Geometry: final body of the model. Coordinates: model frame, mm. A direction names the side the tool comes from. Give positions to 0.01 mm unless a question says otherwise; leave off trailing zeros. Order: outer loops, then holes, each group sorted by start corner. A loop starts at its lowest first (then second) coordinate and runs counter-clockwise, first axis right, second up. Notation, with made-up numbers: (61.5, -14) - (92.5, -14) arc R21 ccw to (92.5, 18) - close; hole circle Ø7 at (33.25, -5). An arc over 180 degrees is marked (long way). Put each result on its own line as item: value. Start each with the question number.
1. Section B-B on x = 4.65. Return the cut outline in (y, z), plus the area to 3 significant figures.
2. Ray query, line 1 along Y through (x, z) = (0, 0.9); line 2 along Z through (x, y) = (1.25, 1.25); line 3 along Z through (x, y) = (0.5, 4.25). Return the intervals inside material, ascending. Write a range as from..to.
3. Set-up query: faces 5 (the flat face through (-1, -1, 1.1)), 6 (the flat face through (1.9, 5, 1)), 7 (the flat face through (-1, -1, 1.33)), 8 (the flat face through (1.9, -5, 1)). Return all of +Z, -Z, +X, -X, +Y, -Y with unobstructed straight access to the full face (end or side cutting, diameter ignored); none if empty.
4. Mould query, pull axis Y, two halves, no side actions, for faces 1 (the flat face through (-1.9, -5, 1)), 2 (the cylindrical face through (-10.94, -1.79, 0.66)), 3 (the cylindrical face through (0, 8.4, 0.7)), 4 (the cylindrical face through (-8.221, 0.135, 0.674)). Classes: pulls with the +Y half, pulls with the -Y half, needs draft (parallel to the pull), parting line crosses it, or undercut.
5. First-contact query: P1, Ø2, axis at x = -4.5, z = 3, coming from the -Y side; P2, Ø4, axis at x = 0, y = 0, coming from the -Z side; P3, Ø1.5, axis at y = 5.5, z = 0.5, coming from the -X side; P4, Ø1.5, axis at x = -9, z = 0.5, coming from the -Y side. Flat tips, straight axial feed; report the tip coordinate or a pass-through.
6. Section A-A on z = 0.8. Count the separate pieces of the cut face and the enclosed holes in it, plus the area to 3 significant figures.
7. Section C-C on z = 3.3. Return the cut outline in (x, y), plus the area to 3 significant figures.
from build123d import *

# Parameters (mm, degrees)
AUFSATZ_LINEAR_AUSTRAGEN1_DEPTH      = 1.33
SKIZZE2_R                            = 3.4
SKIZZE2_R_2                          = 2.3
AUFSATZ_LINEAR_AUSTRAGEN2_DEPTH      = 2.3
AUFSATZ_LINEAR_AUSTRAGEN2_DEPTH_BACK = 1.33
SKIZZE3_R                            = 1.25
SCHNITT_LINEAR_AUSTRAGEN1_DEPTH      = 2.33
SKIZZE4_R                            = 2.35
SCHNITT_LINEAR_AUSTRAGEN2_DEPTH      = 1.1
SKIZZE5_R                            = 0.45
SCHNITT_LINEAR_AUSTRAGEN3_DEPTH      = 2.33
SKIZZE7_W                            = 8.843573308
SKIZZE7_H                            = 7.939116947
SKIZZE7_W_2                          = 8.543023068
SKIZZE7_H_2                          = 6.617341639
SCHNITT_LINEAR_AUSTRAGEN4_DEPTH      = 1.33
VERRUNDUNG1_R                        = 2


with BuildPart() as part:
    # Skizze1 → Aufsatz-Linear austragen1 (new body)
    with BuildSketch(Plane.XY):
        with BuildLine():
            Line((-16.79191458, 1.869621687), (-1.9, 3))
            Line((-1.9, 3), (-1.9, 6.5))
            ThreePointArc((-1.9, 6.5), (0, 8.4), (1.9, 6.5))
            Line((1.9, 6.5), (1.9, 3))
            Line((1.9, 3), (16.79191458, 1.869621687))
            ThreePointArc((16.79191458, 1.869621687), (18.525, 0), (16.79191458, -1.869621687))
            Line((16.79191458, -1.869621687), (1.9, -3))
            Line((1.9, -3), (1.9, -6.5))
            ThreePointArc((1.9, -6.5), (0, -8.4), (-1.9, -6.5))
            Line((-1.9, -6.5), (-1.9, -3))
            Line((-1.9, -3), (-16.79191458, -1.869621687))
            ThreePointArc((-16.79191458, -1.869621687), (-18.525, 0), (-16.79191458, 1.869621687))
        make_face()
    extrude(amount=AUFSATZ_LINEAR_AUSTRAGEN1_DEPTH)

    # Skizze2 → Aufsatz-Linear austragen2 (add, two sides)
    with BuildSketch(Plane.XY.offset(1.33)) as aufsatz_linear_austragen2_sk:
        Circle(SKIZZE2_R)
        Circle(SKIZZE2_R_2, mode=Mode.SUBTRACT)
    extrude(amount=AUFSATZ_LINEAR_AUSTRAGEN2_DEPTH)
    extrude(aufsatz_linear_austragen2_sk.sketch, amount=-AUFSATZ_LINEAR_AUSTRAGEN2_DEPTH_BACK)

    # Skizze3 → Schnitt-Linear austragen1 (cut, through all)
    with BuildSketch(Plane.XY.offset(1.33)):
        Circle(SKIZZE3_R)
    extrude(amount=-SCHNITT_LINEAR_AUSTRAGEN1_DEPTH, mode=Mode.SUBTRACT)

    # Skizze4 → Schnitt-Linear austragen2 (cut)
    with BuildSketch(Plane(origin=(0, 0, 0), x_dir=(-1, 0, 0), z_dir=(0, 0, -1))):
        Circle(SKIZZE4_R)
    extrude(amount=-SCHNITT_LINEAR_AUSTRAGEN2_DEPTH, mode=Mode.SUBTRACT)

    # Skizze5 → Schnitt-Linear austragen3 (cut, through all)
    with BuildSketch(Plane.XY.offset(1.33)):
        with Locations((0, 6.5)):
            Circle(SKIZZE5_R)
        with Locations((-16.65, 0)):
            Circle(SKIZZE5_R)
        with Locations((0, 4.5)):
            Circle(SKIZZE5_R)
        with Locations((-14.65, 0)):
            Circle(SKIZZE5_R)
        with Locations((-12.65, 0)):
            Circle(SKIZZE5_R)
        with Locations((-10.65, 0)):
            Circle(SKIZZE5_R)
        with Locations((-8.65, 0)):
            Circle(SKIZZE5_R)
        with Locations((-6.65, 0)):
            Circle(SKIZZE5_R)
        with Locations((-4.65, 0)):
            Circle(SKIZZE5_R)
        with Locations((0, -4.5)):
            Circle(SKIZZE5_R)
        with Locations((0, -6.5)):
            Circle(SKIZZE5_R)
        with Locations((4.65, 0)):
            Circle(SKIZZE5_R)
        with Locations((6.65, 0)):
            Circle(SKIZZE5_R)
        with Locations((8.65, 0)):
            Circle(SKIZZE5_R)
        with Locations((10.65, 0)):
            Circle(SKIZZE5_R)
        with Locations((12.65, 0)):
            Circle(SKIZZE5_R)
        with Locations((14.65, 0)):
            Circle(SKIZZE5_R)
        with Locations((16.65, 0)):
            Circle(SKIZZE5_R)
    extrude(amount=-SCHNITT_LINEAR_AUSTRAGEN3_DEPTH, mode=Mode.SUBTRACT)

    # Skizze7 → Schnitt-Linear austragen4 (cut)
    with BuildSketch(Plane(origin=(0, 0, 0), x_dir=(-1, 0, 0), z_dir=(0, 0, -1))):
        with Locations((-15.777738742, 0.234488686)):
            Rectangle(SKIZZE7_W, SKIZZE7_H)
        with Locations((15.758609631, 0.140049559)):
            Rectangle(SKIZZE7_W_2, SKIZZE7_H_2)
    extrude(amount=-SCHNITT_LINEAR_AUSTRAGEN4_DEPTH, mode=Mode.SUBTRACT)

    # Verrundung1
    verrundung1_edges = [part.edges().sort_by_distance(p)[0] for p in [
        (11.355952088, -2.282241171, 0.665),
        (11.355952088, 2.282241171, 0.665),
        (-11.487098097, -2.272286467, 0.665),
        (-11.487098097, 2.272286467, 0.665),
    ]]
    fillet(verrundung1_edges, radius=VERRUNDUNG1_R)


solid = part.part
Resolved:
1. outline: (-2.79, 0) - (-0.45, 0) - (-0.45, 1.33) - (-2.79, 1.33) - close; (0.45, 0) - (2.79, 0) - (2.79, 1.33) - (0.45, 1.33) - close
1. area: 6.23 mm^2
2. line 1: -8.4..-6.95, -6.05..-4.95, -4.05..-2.35, 2.35..4.05, 4.95..6.05, 6.95..8.4
2. line 2: 1.1..1.33
2. line 3: 0..1.33
3. face 5: -Z
3. face 6: +Z, -Z, +X, +Y
3. face 7: +Z
3. face 8: +Z, -Z, +X, -Y
4. face 1: needs draft
4. face 2: pulls with the -Y half
4. face 3: pulls with the +Y half
4. face 4: undercut
5. P1: through
5. P2: z = 1.1
5. P3: x = -1.9
5. P4: y = -2.52
6. separate pieces: 1
6. enclosed holes: 13
6. area: 133 mm^2
7. outline: circle Ø6.8 at (0, 0); hole circle Ø4.6 at (0, 0)
7. area: 19.7 mm^2
